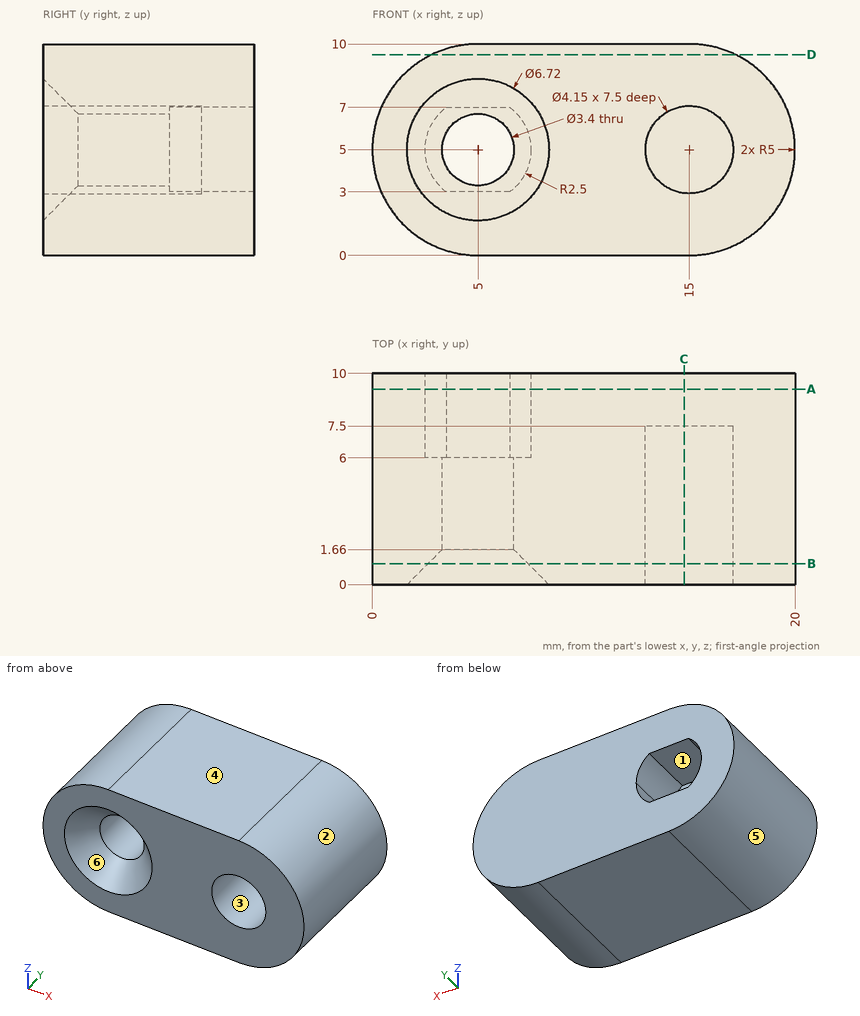
Design review of the part shown in the three views and the two pictorial views. Dimensions are in mm from the part's minimum x, y and z. A direction names the side the tool comes from. Coordinates: 2 decimals unless noted, no trailing zeros. Write each loop counter-clockwise with the first axis right and the second up, starting at its lowest first coordinate (ties: lowest second). Pieces come first, ordered by that corner, then holes.
1) Clearance check with flat-ended pins moving along their axes: pin 1 Ø2 at (y, z) = (3.5, 8.5) entering from +X; pin 2 Ø1 at (y, z) = (6, 8.5) entering from +X; pin 3 Ø4.5 at (x, z) = (5, 5) entering from +Y; pin 4 Ø1.2 at (x, z) = (14.5, 5.5) entering from -Y. State where each tip first meets the part, or that it passes through.
2) The part is to be moulded in two halves that separate along X. For the marked faces 4, 5 and 6, say which applies: pulls with the +X half, pulls with the -X half, needs draft (parallel to the pull), parting line crosses it, or undercut.
3) Machinability: for the marked faces 1, 2 and 3, which of the approach directions +Z, -Z, +X, -X, +Y, -Y give a long, thin tool a straight path to every point of the face, cutting with its end or side? Answer none if there is none.
4) We need section D-D on z = 9.5. State the section outline as (x, y) points.
5) We need section B-B on y = 1. State the section outline as (x, z) points (3 decimals), then the cut area to 3 significant figures.
6) We need section A-A on y = 9.25. State the section outline as (x, z) points.
7) We need section C-C on x = 14.75. State the section outline as (y, z) points, then the cut area to 3 significant figures.
8) To check wall thickness, follow probe 1 along Z at (x, y) = (5, 3.2); probe 2 along Z at (x, y) = (15, 4.25) (3 decimals); probe 3 along X at (y, z) = (2.75, 4). State the ranges of each line that lie inside material, in increasing order.
Answer list:
1. pin 1: stops at x = 19.33
1. pin 2: stops at x = 19
1. pin 3: stops at y = 10
1. pin 4: stops at y = 7.5
2. face 4: needs draft
2. face 5: pulls with the -X half
2. face 6: undercut
3. face 1: +Y
3. face 2: +X, +Y, -Y
3. face 3: -Y
4. outline: (2.82, 0) - (17.18, 0) - (17.18, 10) - (2.82, 10) - close
5. outline: (5, 0) - (15, 0) arc R5 ccw to (15, 10) - (5, 10) arc R5 ccw to start; hole circle Ø4.72 at (5, 5); hole circle Ø4.15 at (15, 5)
5. area: 148 mm2
6. outline: (5, 0) - (15, 0) arc R5 ccw to (15, 10) - (5, 10) arc R5 ccw to start; hole (3.5, 3) - (6.5, 3) arc R2.5 ccw to (6.5, 7) - (3.5, 7) arc R2.5 ccw to start
7. outline: (0, 0) - (10, 0) - (10, 10) - (0, 10) - (0, 7.06) - (7.5, 7.06) - (7.5, 2.94) - (0, 2.94) - close
7. area: 69.1 mm2
8. probe 1: z = 0 to 3.3, 6.7 to 10
8. probe 2: z = 0 to 2.925, 7.075 to 10
8. probe 3: x = 0.1 to 3.63, 6.37 to 13.18, 16.82 to 19.9
